```python
from build123d import *

# Parameters (mm, degrees)
SKETCH3_R           = 9
BOSS_EXTRUDE3_DEPTH = 35
CUT_EXTRUDE1_DEPTH  = 6.5
FILLET1_R           = 1
SKETCH1_R           = 3.05
CUT_EXTRUDE2_DEPTH  = 7
CHAMFER1_SIZE       = 3.05
CHAMFER2_SIZE       = 0.5


with BuildPart() as part:
    # Sketch3 → Boss-Extrude3 (new body)
    with BuildSketch(Plane(origin=(0, 0, 0), x_dir=(1, 0, 0), z_dir=(0, 1, 0))):
        with Locations(Location((0, 0, 0), (0, 0, 270))):
            Circle(SKETCH3_R)
    extrude(amount=BOSS_EXTRUDE3_DEPTH)

    # Sketch4 → Cut-Extrude1 (cut)
    with BuildSketch(Plane(origin=(0, 35, 0), x_dir=(1, 0, 0), z_dir=(0, 1, 0))):
        with BuildLine():
            ThreePointArc((0, -3.25), (5.548097039, -5.548097039), (3.25, 0))
            ThreePointArc((3.25, 0), (5.548097039, 5.548097039), (0, 3.25))
            ThreePointArc((0, 3.25), (-5.548097039, 5.548097039), (-3.25, 0))
            ThreePointArc((-3.25, 0), (-5.548097039, -5.548097039), (0, -3.25))
        make_face()
    extrude(amount=-CUT_EXTRUDE1_DEPTH, mode=Mode.SUBTRACT)

    # Fillet1
    fillet1_edges = [part.edges().sort_by_distance(p)[0] for p in [
        (-3.25, 31.75, 0),
        (0, 31.75, -3.25),
        (3.25, 31.75, 0),
        (0, 31.75, 3.25),
    ]]
    fillet(fillet1_edges, radius=FILLET1_R)

    # Sketch1 → Cut-Extrude2 (cut)
    with BuildSketch(Plane(origin=(0, 0, 0), x_dir=(-1, 0, 0), z_dir=(0, -1, 0))):
        with Locations(Location((0, 0, 0), (0, 0, 90))):
            Circle(SKETCH1_R)
    extrude(amount=-CUT_EXTRUDE2_DEPTH, mode=Mode.SUBTRACT)

    # Chamfer1
    chamfer1_edges = [part.edges().sort_by_distance(p)[0] for p in [
        (0, 7, 3.05),
    ]]
    chamfer(chamfer1_edges, length=CHAMFER1_SIZE)

    # Chamfer2
    chamfer2_edges = [part.edges().sort_by_distance(p)[0] for p in [
        (0, 0, -9),
        (0, 35, -9),
    ]]
    chamfer(chamfer2_edges, length=CHAMFER2_SIZE)


solid = part.part
```
Check sheet for the modelled part. Datum: model origin and axes. Units: mm. A direction names the side the tool comes from. Give positions to 0.01 mm unless a question says otherwise; leave off trailing zeros. Write each loop counter-clockwise with the first axis right and the second up, starting at its lowest first coordinate (ties: lowest second). Pieces come first, ordered by that corner, then holes.
Item 1: Access from +Z, -Z, +X, -X, +Y, -Y to the whole of each face (thin tool, end or side, straight path). Record for faces 1 (the face through (0, 0, 4)), 2 (the face through (5.494, 31.796, 5.601)), 3 (the face through (-1.856, 1.947, 2.42)).
Item 2: Cross-section at A-A (y = 5.5). Enter the section's corners in (x, z).
Item 3: Scan lines: L1, parallel to X at y = 31, z = -5.5; L2, parallel to Y at x = -3.5, z = -2.5. Record each from-to range of solid material in increasing order.
Item 4: Draft check along X on faces 4 (the face through (-6, 35, 1)), 5 (the face through (-5.494, 31.796, -5.601)), 6 (the face through (2.703, 17.262, 8.584)). Enter one of: released by +X, released by -X, zero draft, split by the parting line, or undercut.
Item 5: Gauge pin test, flat ends, axial feed: pin 1 (5 mm diameter, centred on x = -6.5, z = -6, fed in from -Y); pin 2 (4 mm diameter, centred on y = 4, z = 5.5, fed in from +X); pin 3 (6 mm diameter, centred on y = 31, z = -4.5, fed in from +X); pin 4 (4 mm diameter, centred on x = 4.5, y = 5.5, fed in from +Z). Record the tip position at first contact, or that the pin passes through.
Item 6: Cross-section at B-B (y = 22). Enter the section's corners in (x, z).
Report:
1. face 1: +Z, -Z, +X, -X, -Y
1. face 2: +Y
1. face 3: -Y
2. outline: circle Ø18 at (0, 0); hole circle Ø3 at (0, 0)
3. L1: x = -7.12 to -5.6, -0.9 to 0.9, 5.6 to 7.12
3. L2: y = 0 to 28.5
4. face 4: zero draft
4. face 5: undercut
4. face 6: split by the parting line
5. pin 1: stops at y = 0
5. pin 2: stops at x = 8.29
5. pin 3: stops at x = 8.87
5. pin 4: stops at z = 8.65
6. outline: circle Ø18 at (0, 0)
